Geometry check sheet. Reference: the model listing, model coordinates, mm. Face numbers are marked on the shaded views. A direction names the side the tool comes from. Give positions to 0.01 mm unless a question says otherwise; leave off trailing zeros. Loops run counter-clockwise (first coordinate to the right, second up) from the corner with the lowest first, then second, coordinate; pieces in that order, holes last.
1. Cross-section at A-A, the plane z = -13. Record the cut outline in (x, y), plus the area to 3 significant figures.
2. Tool access check on the marked faces 4 and 5. Record the directions out of +Z, -Z, +X, -X, +Y, -Y that give a thin tool (end or side, any length) a straight path to the whole face; none if there is none.
3. Release check for a two-part mould opening along Y. For the marked faces 1, 2 and 3 record: +Y half, -Y half, draft (parallel to the pull), parting line (faces both ways), or undercut.
4. Material ranges on L1, parallel to Z at x = -1.25, y = 4; L2, parallel to Z at x = -4.5, y = -7; L3, parallel to Z at x = 4, y = -3, recorded low to high.
5. Cross-section at C-C, the plane y = -15. Record the cut outline in (x, z).
6. Cross-section at D-D, the plane y = 12.7. Record the cut outline in (x, z) (3 decimals), plus the area to 3 significant figures.
7. Cross-section at B-B, the plane y = 19. Record the cut outline in (x, z).
8. Go/stop test with flat-tipped pins: pin 1 Ø5 at (x, y) = (1.5, 4) entering from -Z; pin 2 Ø4 at (x, z) = (4.5, 62) entering from +Y (3 decimals); pin 3 Ø3 at (x, z) = (2.5, -11) entering from -Y. Record where each tip stops, or that it passes through.
from build123d import *

# Parameters (mm, degrees)
F1_DEPTH = 6.35
F3_DEPTH = 6.35
F4_R     = 5.08
F5_R     = 5.08


with BuildPart() as f1:
    # F0 (on Right) → F1 (new body, symmetric)
    with BuildSketch(Plane.YZ):
        with BuildLine():
            Line((-2.3884117353, 6.5878875691), (-11.3389839483, 9.8456294343))
            ThreePointArc((-11.3389839483, 9.8456294343), (-24.7681294343, 3.5835160517), (-18.5060160517, -9.8456294343))
            Line((-18.5060160517, -9.8456294343), (17.2962728002, -22.876596895))
            ThreePointArc((17.2962728002, -22.876596895), (28.7503201953, -19.9470893959), (30.1830436792, -8.2114803647))
            Line((30.1830436792, -8.2114803647), (-2.8054247121, 55.4675215066))
            ThreePointArc((-2.8054247121, 55.4675215066), (15.9289301948, 80.6613786173), (24.2258585116, 50.3815590934))
            ThreePointArc((24.2258585116, 50.3815590934), (30.7726917058, 37.1897530277), (31.6517846048, 51.8905002135))
            ThreePointArc((31.6517846048, 51.8905002135), (13.495941442, 85.7107429462), (-7.0341769063, 53.2768455539))
            Line((-7.0341769063, 53.2768455539), (25.954291485, -10.4021563174))
            ThreePointArc((25.954291485, -10.4021563174), (25.1728059483, -16.8033976072), (18.9251437328, -18.4013107885))
            Line((18.9251437328, -18.4013107885), (-16.8771451191, -5.3703433278))
            ThreePointArc((-16.8771451191, -5.3703433278), (-20.2928433278, 1.9546451191), (-12.9678548809, 5.3703433278))
            Line((-12.9678548809, 5.3703433278), (-4.0172826679, 2.1126014626))
            ThreePointArc((-4.0172826679, 2.1126014626), (-0.9652041484, 3.5358090496), (-2.3884117353, 6.5878875691))
        make_face()
    extrude(amount=F1_DEPTH, both=True)

    # F2 (on Right) → F3 (join, symmetric)
    with BuildSketch(Plane.YZ):
        with BuildLine():
            Line((25.954291485, -10.4021563174), (23.3565733209, -5.3876737451))
            ThreePointArc((23.3565733209, -5.3876737451), (23.915643926, -12.8393677138), (18.9251437328, -18.4013107885))
            ThreePointArc((18.9251437328, -18.4013107885), (25.1728059483, -16.8033976072), (25.954291485, -10.4021563174))
        make_face()
        with BuildLine():
            ThreePointArc((30.1625, 63.5), (12.7, 80.9625), (-4.7625, 63.5))
            ThreePointArc((-4.7625, 63.5), (12.7, 77.9349299335), (30.1625, 63.5))
        make_face()
    extrude(amount=F3_DEPTH, both=True)

    # F4
    f4_edges = [f1.edges().sort_by_distance(p)[0] for p in [
        (0, 31.651785, 51.8905),
    ]]
    fillet(f4_edges, radius=F4_R)

    # F5
    f5_edges = [f1.edges().sort_by_distance(p)[0] for p in [
        (0, 18.925144, -18.401311),
    ]]
    fillet(f5_edges, radius=F5_R)


solid = f1.part
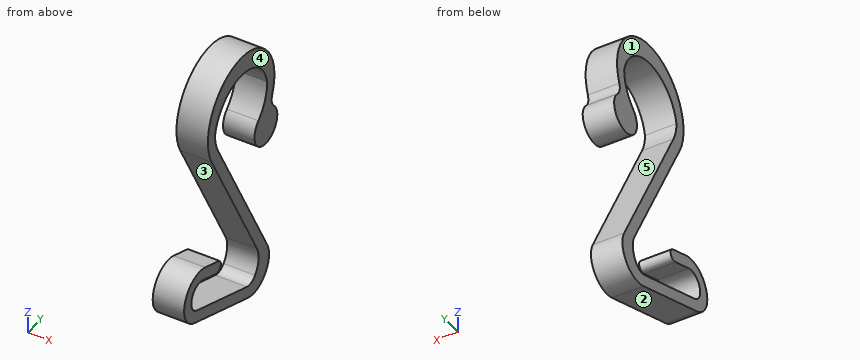
Result:
1. outline: (-6.35, -9.84) - (6.35, -9.84) - (6.35, 4.09) - (-6.35, 4.09) - close; (-6.35, 23.86) - (6.35, 23.86) - (6.35, 31.36) - (-6.35, 31.36) - close
1. area: 272 mm2
2. face 4: +Z, -Z, +X, +Y, -Y
2. face 5: +X, -X
3. face 1: draft
3. face 2: -Y half
3. face 3: undercut
4. L1: z = -18.04 to -12.97, 31.98 to 42.33, 75.66 to 83.95
4. L2: z = -14.03 to -8.97, 3.2 to 8.27, 53.21 to 73.79
4. L3: z = -15.49 to -10.42, 1.98 to 6.81, 45.49 to 55.85, 68.5 to 79.23
5. outline: (-6.35, -11.12) - (6.35, -11.12) - (6.35, -6.05) - (-6.35, -6.05) - close; (-6.35, 5.71) - (6.35, 5.71) - (6.35, 10.48) - (-6.35, 10.48) - close
6. outline: (-6.35, -21.204) - (6.35, -21.204) - (6.35, -16.136) - (-6.35, -16.136) - close; (-6.35, 15.183) - (6.35, 15.183) - (6.35, 25.537) - (-6.35, 25.537) - close; (-6.35, 77.935) - (6.35, 77.935) - (6.35, 85.725) - (-6.35, 85.725) - close
6. area: 295 mm2
7. outline: (-6.35, -23.34) - (6.35, -23.34) - (6.35, -17.75) - (-6.35, -17.75) - close; (-6.35, 3.02) - (6.35, 3.02) - (6.35, 13.38) - (-6.35, 13.38) - close; (-6.35, 76.78) - (6.35, 76.78) - (6.35, 84.81) - (-6.35, 84.81) - close
8. pin 1: stops at z = -18.95
8. pin 2: stops at y = 34.925
8. pin 3: stops at y = -19.34
